Verification items for the finished model (mm, model axes). Round coordinates to 2 decimals unless told otherwise and drop trailing zeros. Write each loop counter-clockwise with the first axis right and the second up, starting at its lowest first coordinate (ties: lowest second). Pieces come first, ordered by that corner, then holes.
from build123d import *

# Parameters (mm, degrees)
SKETCH_1_W                  = 80
SKETCH_1_H                  = 56
SKETCH_1_R                  = 13
EXTRUDE_1_DEPTH             = 4
SKETCH_2_R                  = 2
CUT_EXTRUDE_1_DEPTH         = 100
PATTERN_LINEAR_1_COUNT      = 2
PATTERN_LINEAR_1_PITCH      = 44
PATTERN_LINEAR_1_COUNT_DIR2 = 2
PATTERN_LINEAR_1_PITCH_DIR2 = 50
SKETCH_3_R                  = 3
CUT_EXTRUDE_2_DEPTH         = 50


with BuildPart() as part:
    # 草图1 → 凸台-拉伸1 (new body)
    with BuildSketch(Plane.XY):
        with Locations((0, 7)):
            Rectangle(SKETCH_1_W, SKETCH_1_H)
        with Locations((0, 7)):
            Circle(SKETCH_1_R, mode=Mode.SUBTRACT)
    extrude(amount=EXTRUDE_1_DEPTH)

    # 草图2 → 切除-拉伸1 (cut)
    with BuildSketch(Plane.XY.offset(4)):
        with Locations((-25, -15)):
            Circle(SKETCH_2_R)
    cut_extrude_1 = extrude(amount=-CUT_EXTRUDE_1_DEPTH, mode=Mode.SUBTRACT)

    # 阵列(线性)1: Cut-Extrude 1 2 × 2
    with Locations(*[(j * PATTERN_LINEAR_1_PITCH_DIR2, i * PATTERN_LINEAR_1_PITCH, 0) for i in range(PATTERN_LINEAR_1_COUNT) for j in range(PATTERN_LINEAR_1_COUNT_DIR2) if (i, j) != (0, 0)]):
        add(cut_extrude_1, mode=Mode.SUBTRACT)

    # 草图3 → 切除-拉伸2 (cut)
    with BuildSketch(Plane.XY.offset(4)):
        with Locations((24.051141157, 7)):
            Circle(SKETCH_3_R)
        with Locations((-23.948858843, 7)):
            Circle(SKETCH_3_R)
    extrude(amount=-CUT_EXTRUDE_2_DEPTH, mode=Mode.SUBTRACT)


solid = part.part
Q1. Sectioned sample at C-C (x = 25). Enter the section's corners in (y, z).
Recorded:
outline: (-21, 0) - (-17, 0) - (-17, 4) - (-21, 4) - close; (-13, 0) - (4.15, 0) - (4.15, 4) - (-13, 4) - close; (9.85, 0) - (27, 0) - (27, 4) - (9.85, 4) - close; (31, 0) - (35, 0) - (35, 4) - (31, 4) - close
Q2. Sectioned sample at A-A (x = 5). Enter the section's corners in (y, z), plus the area to 3 significant figures.
Recorded:
outline: (-21, 0) - (-5, 0) - (-5, 4) - (-21, 4) - close; (19, 0) - (35, 0) - (35, 4) - (19, 4) - close
area: 128 mm2
Q3. Sectioned sample at D-D (y = -15). Enter the section's corners in (x, z).
Recorded:
outline: (-40, 0) - (-27, 0) - (-27, 4) - (-40, 4) - close; (-23, 0) - (23, 0) - (23, 4) - (-23, 4) - close; (27, 0) - (40, 0) - (40, 4) - (27, 4) - close
Q4. Release check for a two-part mould opening along X. For faces 1 (the cylindrical face through (-10.316, -0.91, 1.972)), 2 (the flat face through (-1, 35, 2)), 3 (the flat face through (40, 7, 2)) record: released by +X, released by -X, zero draft, split by the parting line, or undercut.
Recorded:
face 1: undercut
face 2: zero draft
face 3: released by +X
Q5. Sectioned sample at B-B (y = 7). Enter the section's corners in (x, z), plus the area to 3 significant figures.
Recorded:
outline: (-40, 0) - (-26.95, 0) - (-26.95, 4) - (-40, 4) - close; (-20.95, 0) - (-13, 0) - (-13, 4) - (-20.95, 4) - close; (13, 0) - (21.05, 0) - (21.05, 4) - (13, 4) - close; (27.05, 0) - (40, 0) - (40, 4) - (27.05, 4) - close
area: 168 mm2
Q6. Material ranges on line 1 along X through (y, z) = (-13.5, 1); line 2 along X through (y, z) = (-14, 1.35); line 3 along Y through (x, z) = (-25, 1.4), recorded low to high.
Recorded:
line 1: x = -40 to -26.32, -23.68 to 23.68, 26.32 to 40
line 2: x = -40 to -26.73, -23.27 to 23.27, 26.73 to 40
line 3: y = -21 to -17, -13 to 4.19, 9.81 to 27, 31 to 35
